Could you check a few things on this drawing? It's one solid part, dimensions in mm from its lowest x, y, z. A direction names the side the tool comes from. Coordinates: 2 decimals unless noted, no trailing zeros. Write each loop counter-clockwise with the first axis right and the second up, starting at its lowest first coordinate (ties: lowest second). Pieces come first, ordered by that corner, then holes. Notation, with made-up numbers: M 45,62 L 92,62 A19 cw 92,84 Z; hole C -24,80 d9. An arc over 180 degrees is marked long. Use a Markdown table: item, result.
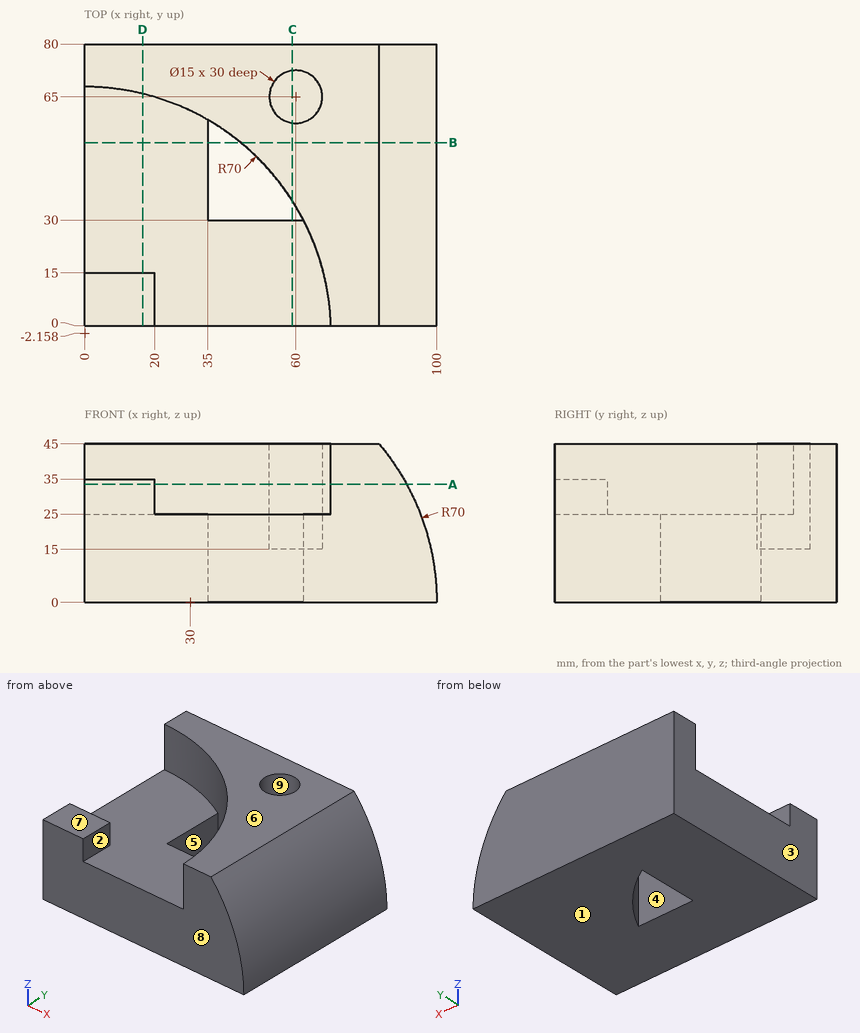
1. Suppose I cut it at B-B on y = 52. Write out the boundary of the cut face in (x, z).
Answers follow:
| item | result |
|---|---|
| outline | M 0,0 L 35,0 L 35,25 L 0,25 Z; M 44.35,0 L 100,0 A70 ccw 83.62,45 L 44.35,45 Z |
2. I need wall thicknesses on probe 1 along Y at (x, z) = (60, 23); probe 2 along Z at (x, y) = (18, 45); probe 3 along Y at (x, z) = (60, 34). Which ranges of each line are inside material? Lowest first, please.
Answers follow:
| item | result |
|---|---|
| probe 1 | y = 0 to 30, 33.9 to 57.5, 72.5 to 80 |
| probe 2 | z = 0 to 25 |
| probe 3 | y = 33.9 to 57.5, 72.5 to 80 |
3. Suppose I cut it at C-C on x = 59. Write out the boundary of the cut face in (y, z).
Answers follow:
| item | result |
|---|---|
| outline | M 0,0 L 30,0 L 30,25 L 0,25 Z; M 35.51,0 L 80,0 L 80,45 L 72.43,45 L 72.43,15 L 57.57,15 L 57.57,45 L 35.51,45 Z |
4. Suppose I cut it at D-D on x = 16.5. Write out the boundary of the cut face in (y, z), and give its area (3 significant figures).
Answers follow:
| item | result |
|---|---|
| outline | M 0,0 L 80,0 L 80,45 L 65.87,45 L 65.87,25 L 15,25 L 15,35 L 0,35 Z |
| area | 2,430 mm2 |
5. Which directions (+Z, -Z, +X, -X, +Y, -Y) give clear straight access to the entire face, cutting with the end or side of a thin tool? Please do the marked faces 5, 6, 7, 8 and 9.
Answers follow:
| item | result |
|---|---|
| face 5 | +Z, -Z |
| face 6 | +Z, +X, -X, +Y, -Y |
| face 7 | +Z, -X, -Y |
| face 8 | +Z, -Z, +X, -X, -Y |
| face 9 | +Z |
6. Will these pins go through, and if not, where does the flat tip stop? pin 1 Ø8 at (x, z) = (22, 40) entering from -Y; pin 2 Ø5 at (x, z) = (48, 28.5) entering from -Y; pin 3 Ø4.5 at (x, y) = (59, 63) entering from +Z.
Answers follow:
| item | result |
|---|---|
| pin 1 | stops at y = 62.83 |
| pin 2 | stops at y = 46.32 |
| pin 3 | stops at z = 15 |
7. We'd pull the mould along X, two halves only. Please class the marked faces 1, 2, 3 and 4: +X half, -X half, draft (parallel to the pull), parting line (faces both ways), or undercut.
Answers follow:
| item | result |
|---|---|
| face 1 | draft |
| face 2 | undercut |
| face 3 | -X half |
| face 4 | undercut |
8. Suppose I cut it at A-A on z = 33.5. Write out the boundary of the cut face in (x, y).
Answers follow:
| item | result |
|---|---|
| outline | M 0,0 L 20,0 L 20,15 L 0,15 Z; M 0,67.84 A70 cw 69.97,0 L 91.46,0 L 91.46,80 L 0,80 Z; hole C 60,65 d15 |
